Here's how the part is built. I have some questions about the finished solid (model axes, mm). Face numbers are marked on the shaded views. A direction names the side the tool comes from. Round coordinates to 2 decimals unless told otherwise and drop trailing zeros. Order: outer loops, then holes, each group sorted by start corner. A loop starts at its lowest first (then second) coordinate and runs counter-clockwise, first axis right, second up. Notation, with made-up numbers: (77.5, -10) -> (108.5, -10) arc R29 ccw to (108.5, 17) -> close; hole circle Ø9 at (35, 7). An arc over 180 degrees is marked (long way). Answer in a Markdown table with one row per item.
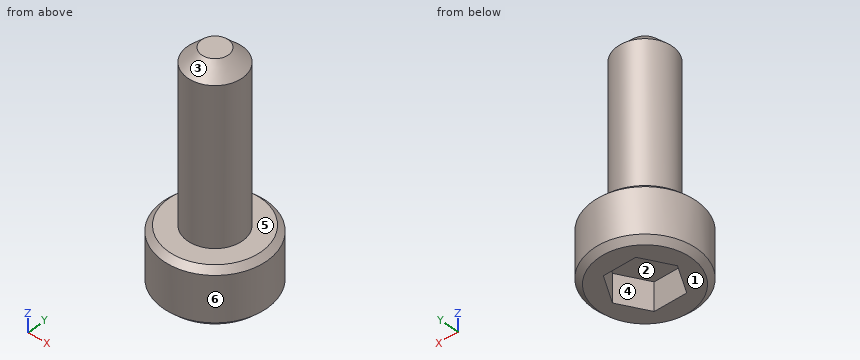
```python
from build123d import *

# Parameters (mm, degrees)
SKETCH3_R           = 1.835
BOSS_EXTRUDE1_DEPTH = 2
SKETCH4_R           = 0.97
BOSS_EXTRUDE2_DEPTH = 6
CHAMFER1_SIZE       = 0.5
CUT_EXTRUDE1_DEPTH  = 1
CHAMFER2_SIZE       = 0.2


with BuildPart() as part:
    # Sketch3 → Boss-Extrude1 (new body)
    with BuildSketch(Plane.XY):
        Circle(SKETCH3_R)
    extrude(amount=BOSS_EXTRUDE1_DEPTH)

    # Sketch4 → Boss-Extrude2 (add)
    with BuildSketch(Plane.XY.offset(2)):
        Circle(SKETCH4_R)
    extrude(amount=BOSS_EXTRUDE2_DEPTH)

    # Chamfer1
    chamfer1_edges = [part.edges().sort_by_distance(p)[0] for p in [
        (-0.97, 0, 8),
    ]]
    chamfer(chamfer1_edges, length=CHAMFER1_SIZE)

    # Sketch5 → Cut-Extrude1 (cut)
    with BuildSketch(Plane(origin=(0, 0, 0), x_dir=(-1, 0, 0), z_dir=(0, 0, -1))):
        Polygon((1.145251225, 0), (0.572625613, 0.991816655), (-0.572625613, 0.991816655), (-1.145251225, 0), (-0.572625613, -0.991816655), (0.572625613, -0.991816655), align=None)
    extrude(amount=-CUT_EXTRUDE1_DEPTH, mode=Mode.SUBTRACT)

    # Chamfer2
    chamfer2_edges = [part.edges().sort_by_distance(p)[0] for p in [
        (-1.835, 0, 0),
        (-1.835, 0, 2),
    ]]
    chamfer(chamfer2_edges, length=CHAMFER2_SIZE)


solid = part.part
```
1. Please list where these lines run through material, in increasing order: line 1 along Z through (x, y) = (-0.35, -1.45); line 2 along Z through (x, y) = (-0.2, 0.2); line 3 along Y through (x, z) = (1.1, 0.5).
Numbers:
| item | result |
|---|---|
| line 1 | z = 0 to 2 |
| line 2 | z = 1 to 8 |
| line 3 | y = -1.47 to -0.08, 0.08 to 1.47 |
2. We'd pull the mould along X, two halves only. Please class the marked faces 1, 2 and 3: released by +X, released by -X, zero draft, split by the parting line, or undercut.
Numbers:
| item | result |
|---|---|
| face 1 | zero draft |
| face 2 | undercut |
| face 3 | split by the parting line |
3. For the marked faces 4, 5 and 6, which set-ups out of +Z, -Z, +X, -X, +Y, -Y let a thin tool reach every point of the face, with its end or its side?
Numbers:
| item | result |
|---|---|
| face 4 | -Z |
| face 5 | +Z |
| face 6 | +Z, -Z |
4. Suppose I cut it at A-A on x = 0. Write out the boundary of the cut face in (y, z) (3 decimals), then the cut area to 3 significant figures.
Numbers:
| item | result |
|---|---|
| outline | (-1.835, 0.2) -> (-1.635, 0) -> (-0.992, 0) -> (-0.992, 1) -> (0.992, 1) -> (0.992, 0) -> (1.635, 0) -> (1.835, 0.2) -> (1.835, 1.8) -> (1.635, 2) -> (0.97, 2) -> (0.97, 7.5) -> (0.47, 8) -> (-0.47, 8) -> (-0.97, 7.5) -> (-0.97, 2) -> (-1.635, 2) -> (-1.835, 1.8) -> close |
| area | 16.7 mm2 |
5. For pin 1 Ø1 at (y, z) = (1, 2) entering from +X, with a flat end and sliding along its axis, tell me the tip position at first contact or that it passes through.
Numbers:
| item | result |
|---|---|
| pin 1 | stops at x = 1.75 |
6. Suppose I cut it at B-B on z = 5.5. Write out the boundary of the cut face in (x, y), then the cut area to 3 significant figures.
Numbers:
| item | result |
|---|---|
| outline | circle Ø1.94 at (0, 0) |
| area | 2.96 mm2 |
